from build123d import *

# Parameters (mm, degrees)
SKETCH1_W             = 50
SKETCH1_H             = 3
SOLARPANET_DEPTH      = 27.5
FILLET1_R             = 2
FILLET2_R             = 1.5
SKETCH2_W             = 50
SKETCH2_H             = 5
BACKSUPPORT_DEPTH     = 2
SKETCH3_R             = 6.5
SKETCH3_R_2           = 5
SUPPORTRING_DEPTH     = 5
HOLE_START            = -5
SKETCH4_R             = 5
HOLE_4_JOYSTICK_DEPTH = 5
FILLET4_R             = 0.5


with BuildPart() as part:
    # Sketch1 → SolarPanet (new, symmetric)
    with BuildSketch(Plane.XY):
        with Locations((25, 1.5)):
            Rectangle(SKETCH1_W, SKETCH1_H)
    extrude(amount=SOLARPANET_DEPTH, both=True)

    # Fillet1
    fillet1_edges = [part.edges().sort_by_distance(p)[0] for p in [
        (50, 1.5, 27.5),
        (0, 1.5, 27.5),
        (50, 1.5, -27.5),
        (0, 1.5, -27.5),
    ]]
    fillet(fillet1_edges, radius=FILLET1_R)

    # Fillet2
    fillet2_edges = [part.edges().sort_by_distance(p)[0] for p in [
        (0, 3, 0),
        (25, 3, -27.5),
        (25, 3, 27.5),
        (50, 3, 0),
        (0.585786438, 3, 26.914213562),
        (49.414213562, 3, 26.914213562),
        (49.414213562, 3, -26.914213562),
        (0.585786438, 3, -26.914213562),
    ]]
    fillet(fillet2_edges, radius=FILLET2_R)

    # Sketch2 → BackSupport (add)
    with BuildSketch(Plane.XZ):
        with Locations((25, 0)):
            Rectangle(SKETCH2_W, SKETCH2_H)
    extrude(amount=BACKSUPPORT_DEPTH)

    # Sketch3 → SupportRing (add)
    with BuildSketch(Plane.XZ):
        with Locations((25, 0)):
            Circle(SKETCH3_R)
        with Locations((25, 0)):
            Circle(SKETCH3_R_2, mode=Mode.SUBTRACT)
    extrude(amount=SUPPORTRING_DEPTH)

    # Sketch4 → Hole 4 Joystick (cut)
    with BuildSketch(Plane.XZ.offset(5).offset(HOLE_START)):
        with Locations((25, 0)):
            Circle(SKETCH4_R)
    extrude(amount=HOLE_4_JOYSTICK_DEPTH, mode=Mode.SUBTRACT)

    # Sketch5 → Round Cut 4 Joystick (revolve, cut)
    with BuildSketch(Plane.XY, mode=Mode.PRIVATE) as round_cut_4_joystick_sk:
        with BuildLine():
            Line((25, -1.64), (30, -1.64))
            ThreePointArc((30, -1.64), (31.43, -3.07), (30, -4.5))
            Line((30, -4.5), (25, -4.5))
            Line((25, -4.5), (25, -1.64))
        make_face()
    revolve(round_cut_4_joystick_sk.sketch.rotate(Axis((25, 10.438378753, 0), (0, -1, 0)), 22.619864948), axis=Axis((25, 10.438378753, 0), (0, -1, 0)), mode=Mode.SUBTRACT)

    # Fillet4
    fillet4_edges = [part.edges().sort_by_distance(p)[0] for p in [
        (20, -5, 0),
        (18.5, -5, 0),
    ]]
    fillet(fillet4_edges, radius=FILLET4_R - 0.0001)  # a hair under: the kernel refuses the full size


solid = part.part
Work out the finished part from the listing and answer in its coordinate system (mm). A direction names the side the tool comes from. Give positions to 0.01 mm unless a question says otherwise; leave off trailing zeros. Write each loop counter-clockwise with the first axis right and the second up, starting at its lowest first coordinate (ties: lowest second). Pieces come first, ordered by that corner, then holes. Notation, with made-up numbers: (50, 43.25) - (84, 43.25) arc R3 cw to (84, 47.25) - close; hole circle Ø11 at (47.5, -16). An arc over 180 degrees is marked (long way). One line per item, written item: value. Start each with the question number.
1. Find section A-A (x = 42). Write down the section's boundary in (y, z), then the cut area to 3 significant figures.
2. For faces 1 (the flat face through (9, -1, -2.5)), 2 (the cylindrical face through (0.43, 2.55, -0.36)), 3 (the cylindrical face through (18.506, -2.219, 0.286)), 4 (the flat face through (9, -1, 2.5)), 5 (the flat face through (40, -1, -2.5)), determine the directions among +Z, -Z, +X, -X, +Y, -Y from which every point of the face is accessible in a straight line to the end or side of a thin tool.
3. Consider probe 1 along X at (y, z) = (-0.9, 0); probe 2 along Z at (x, y) = (25, -1); probe 3 along Z at (x, y) = (14, -0.75). Determine where each line is inside the solid, lowest interval first.
4. Given pin 1 (2 mm diameter, centred on x = 34, z = 9, fed in from -Y); pin 2 (0.6 mm diameter, centred on x = 7, y = -1.5, fed in from -Z); pin 3 (8 mm diameter, centred on x = 27, z = -1.5, fed in from -Y); pin 4 (0.6 mm diameter, centred on x = 9.5, y = -1.5, fed in from +Z), each flat-ended and moving along its own axis, determine where each tip first touches the part or whether it passes through.
5. Find section C-C (z = 7.5). Write down the section's boundary in (x, y).
Geometry results:
1. outline: (-2, -2.5) - (0, -2.5) - (0, -27.5) - (1.5, -27.5) arc R1.5 ccw to (3, -26) - (3, 26) arc R1.5 ccw to (1.5, 27.5) - (0, 27.5) - (0, 2.5) - (-2, 2.5) - close
1. area: 174 mm2
2. face 1: -Z, -X, -Y
2. face 2: +Z, -Z, -X, +Y
2. face 3: -Y
2. face 4: +Z, -X, -Y
2. face 5: -Z, +X, -Y
3. probe 1: 0 to 20, 30 to 50
3. probe 2: -6.5 to -5, 5 to 6.5
3. probe 3: -2.5 to 2.5
4. pin 1: y = 0
4. pin 2: z = -2.5
4. pin 3: y = -5
4. pin 4: z = 2.5
5. outline: (0, 0) - (50, 0) - (50, 1.5) arc R1.5 ccw to (48.5, 3) - (1.5, 3) arc R1.5 ccw to (0, 1.5) - close
